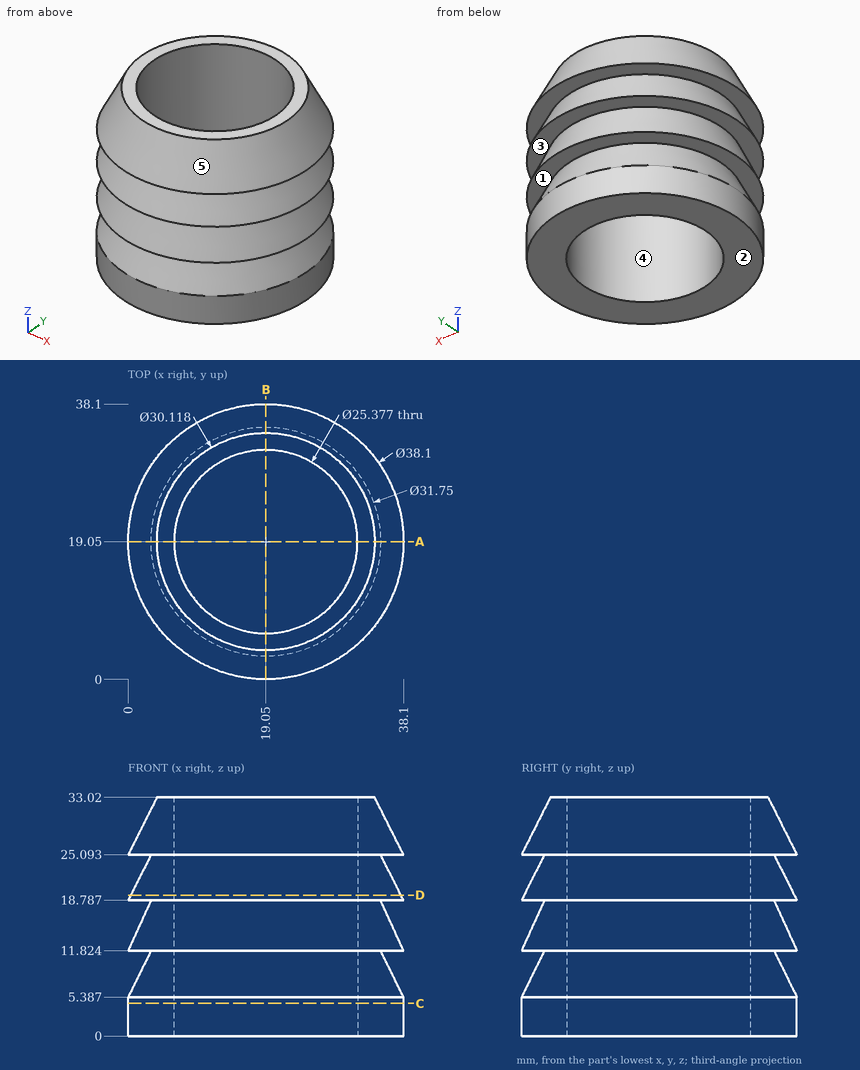
Study the drawing (mm; zero at the part's minimum x, y, z) and answer. A direction names the side the tool comes from. Give positions to 0.01 mm unless a question says otherwise; leave off trailing zeros. Loops run counter-clockwise (first coordinate to the right, second up) from the corner with the lowest first, then second, coordinate; pieces in that order, holes last. Notation, with made-up numbers: (23.25, 71.25) -> (61.25, 71.25) arc R16 ccw to (61.25, 89.25) -> close; hole circle Ø10 at (-28, 55). An arc over 180 degrees is marked (long way). Write item = value, one per line. Start each with the question number.
(1) Which of the six approach directions +Z, -Z, +X, -X, +Y, -Y give full straight-line access (tool end or side, diameter ignored) to the marked faces 1 and 2?
(2) Given pin 1 Ø1 at (y, z) = (28.5, 26.5) entering from -X; pin 2 Ø12 at (x, z) = (16, 18) entering from -Y; pin 3 Ø1.5 at (x, z) = (22, 18) entering from -Y (1 decimal), each flat-ended and moving along its own axis, determine where each tip first touches the part or whether it passes through.
(3) Find the intervals of material crossed by probe 1 along X at (y, z) = (19, 4); probe 2 along X at (y, z) = (26, 29.5) (1 decimal); probe 3 along Y at (x, z) = (10.5, 29) (1 decimal), in increasing order. Write a range as from..to.
(4) Find section A-A on y = 19.05. Give the vertices of the cut face in (x, z) (1 decimal), and give its area (3 significant figures).
(5) Find section C-C on z = 4.5. Give the vertices of the cut face in (x, y).
(6) The mould has two halves that part along X. Classify the marked faces 3, 4 and 5: +X half, -X half, draft (parallel to the pull), parting line (faces both ways), or undercut.
(7) Find section D-D on z = 19.5. Give the vertices of the cut face in (x, y).
From the geometry:
q1.face_1 = none
q1.face_2 = -Z, +X, -X, +Y, -Y
q2.pin_1 = 2.92
q2.pin_2 = 0
q2.pin_3 = 2.7
q3.probe_1 = 0..6.36, 31.74..38.1
q3.probe_2 = 3.7..8.4, 29.7..34.4
q3.probe_3 = 4.3..9.7, 28.4..33.8
q4.outline = (0, 0) -> (6.4, 0) -> (6.4, 33) -> (4, 33) -> (0, 25.1) -> (3.2, 25.1) -> (0, 18.8) -> (3.2, 18.8) -> (0, 11.8) -> (3.2, 11.8) -> (0, 5.4) -> close; (31.7, 0) -> (38.1, 0) -> (38.1, 5.4) -> (34.9, 11.8) -> (38.1, 11.8) -> (34.9, 18.8) -> (38.1, 18.8) -> (34.9, 25.1) -> (38.1, 25.1) -> (34.1, 33) -> (31.7, 33) -> close
q4.area = 326 mm^2
q5.outline = circle Ø38.1 at (19.05, 19.05); hole circle Ø25.38 at (19.05, 19.05)
q6.face_3 = draft
q6.face_4 = undercut
q6.face_5 = parting line
q7.outline = circle Ø37.38 at (19.05, 19.05); hole circle Ø25.38 at (19.05, 19.05)
